from build123d import *

# Parameters (mm, degrees)
BOSS_EXTRUDE1_DEPTH = 2


with BuildPart() as part:
    # Sketch2 → Boss-Extrude1 (new body)
    with BuildSketch(Plane(origin=(0, 0, 0), x_dir=(1, 0, 0), z_dir=(0, 1, 0))):
        Polygon((17.5, 22.5), (22.5, 22.5), (32.5, 11.25), (22.5, 0), (38.5, -11.25), (22.5, -22.5), (17.5, -22.5), (-17.5, -22.5), (-17.5, 22.5), align=None)
        Polygon((17.5, 17.5), (20.254669678, 17.5), (25.810225234, 11.25), (17.261983906, 1.633228506), (15.039761683, 1.633228506), (-9.960238317, 1.633228506), (0.039761683, -3.366771494), (15.039761683, -3.366771494), (18.595317239, -3.366771494), (29.807020003, -11.25), (20.918131114, -17.5), (17.5, -17.5), (-12.5, -17.5), (-12.5, 17.5), align=None, mode=Mode.SUBTRACT)
    extrude(amount=BOSS_EXTRUDE1_DEPTH)


solid = part.part
For this review, take the finished solid that the model builds, in its own axes (mm). A direction names the side the tool comes from. Round coordinates to 2 decimals unless told otherwise and drop trailing zeros. Order: outer loops, then holes, each group sorted by start corner. A loop starts at its lowest first (then second) coordinate and runs counter-clockwise, first axis right, second up. Notation, with made-up numbers: M -38,41 L 18,41 A37 cw 18,77 Z; hole C 41,89.25 d4. An arc over 180 degrees is marked long. Use a Markdown table: item, result. Add a question column.
Item 1: Add section A-A, the plane y = 0.3. Give the boundary of the cut face in (x, z).
Item 2: To check wall thickness, follow line 1 along Z through (x, y) = (2, 1.6); line 2 along Z through (x, y) = (-11, 0.15); line 3 along Z through (x, y) = (-1, 0.4). State the ranges of each line that lie inside material, in increasing order.
Item 3: Add section B-B, the plane x = 24. Give the boundary of the cut face in (y, z).
Item 4: Mouldability with a two-part tool opening along Z and no side actions: class faces 4 (the flat face through (30.61, 0.99, 16.8)), 5 (the flat face through (-17.5, 1, 0)), 6 (the flat face through (9, 1, 3.367)) as released by +Z, released by -Z, zero draft, split by the parting line, or undercut.
Item 5: Tool access review of faces 1 (the flat face through (2, 1, 22.5)), 2 (the flat face through (30.39, 0.99, 5.55)), 3 (the flat face through (-12.5, 1, 0)): name each direction out of +Z, -Z, +X, -X, +Y, -Y from which nothing blocks a thin tool from reaching the whole face with its end or side.
Item 6: Add section C-C, the plane z = 7.5. Give the boundary of the cut face in (x, y).
Item 7: Insertion check: pin 1 (1 mm diameter, centred on y = 1, z = -8, fed in from +X); pin 2 (12 mm diameter, centred on x = 30.5, z = 12, fed in from -Y). Each pin has a flat end and moves straight along its axis. Give the tip position at first contact, or say it passes through.
Item 8: Add section D-D, the plane x = -7. Give the boundary of the cut face in (y, z), then the cut area to 3 significant figures.
Geometry results:
| question | item | result |
|---|---|---|
| 1 | outline | M -17.5,-22.5 L 22.5,-22.5 L 32.5,-11.25 L 22.5,0 L 38.5,11.25 L 22.5,22.5 L -17.5,22.5 Z; hole M -12.5,-17.5 L 20.25,-17.5 L 25.81,-11.25 L 17.26,-1.63 L -9.96,-1.63 L 0.04,3.37 L 18.6,3.37 L 29.81,11.25 L 20.92,17.5 L -12.5,17.5 Z |
| 2 | line 1 | z = -22.5 to -17.5, -1.63 to 3.37, 17.5 to 22.5 |
| 2 | line 2 | z = -22.5 to -17.5, 17.5 to 22.5 |
| 2 | line 3 | z = -22.5 to -17.5, -1.63 to 2.85, 17.5 to 22.5 |
| 3 | outline | M 0,-20.81 L 2,-20.81 L 2,-13.29 L 0,-13.29 Z; M 0,-9.21 L 2,-9.21 L 2,-1.69 L 0,-1.69 Z; M 0,1.05 L 2,1.05 L 2,7.17 L 0,7.17 Z; M 0,15.33 L 2,15.33 L 2,21.45 L 0,21.45 Z |
| 4 | face 4 | released by +Z |
| 4 | face 5 | zero draft |
| 4 | face 6 | undercut |
| 5 | face 1 | +Z, +X, -X, +Y, -Y |
| 5 | face 2 | +X, +Y, -Y |
| 5 | face 3 | +Y, -Y |
| 6 | outline | M -17.5,0 L -12.5,0 L -12.5,2 L -17.5,2 Z; M 24.47,0 L 33.17,0 L 33.17,2 L 24.47,2 Z |
| 7 | pin 1 | stops at x = 30.06 |
| 7 | pin 2 | stops at y = 0 |
| 8 | outline | M 0,-22.5 L 2,-22.5 L 2,-17.5 L 0,-17.5 Z; M 0,-1.63 L 2,-1.63 L 2,-0.15 L 0,-0.15 Z; M 0,17.5 L 2,17.5 L 2,22.5 L 0,22.5 Z |
| 8 | area | 23.0 mm² |
